```python
from build123d import *

# Parameters (mm, degrees)
SKETCH015_R            = 14.2875
SKETCH015_R_2          = 12.7
PAD015_DEPTH           = 29.21
SKETCH016_R            = 16.66875
SKETCH016_R_2          = 12.7
PAD016_DEPTH           = 12.7
SKETCH014_R            = 3.571875
PAD014_DEPTH           = 13
SKETCH013_R            = 34.925
SKETCH013_R_2          = 14.2875
PAD013_DEPTH           = 12.7
CUT006_PLACEMENT_ANGLE = 60
CUT007_PLACEMENT_ANGLE = 60
CUT008_PLACEMENT_ANGLE = 60
CUT009_PLACEMENT_ANGLE = 60
CUT010_PLACEMENT_ANGLE = 60


with BuildPart() as body015:
    # Sketch015 → Pad015 (new body)
    with BuildSketch(Plane.XZ):
        Circle(SKETCH015_R)
        Circle(SKETCH015_R_2, mode=Mode.SUBTRACT)
    extrude(amount=PAD015_DEPTH)


with BuildPart() as body015_1:
    # Body015 placement: moved
    add(body015.part.moved(Location((0, -0.16, 0))))


with BuildPart() as body016:
    # Sketch016 → Pad016 (new body)
    with BuildSketch(Plane.XZ):
        Circle(SKETCH016_R)
        Circle(SKETCH016_R_2, mode=Mode.SUBTRACT)
    extrude(amount=PAD016_DEPTH)


with BuildPart() as body016_1:
    # Body016 placement: moved
    add(body016.part.moved(Location((0, -29.37, 0))))


with BuildPart() as body014:
    # Sketch014 → Pad014 (new body)
    with BuildSketch(Plane.XZ):
        with Locations((0, 29.36875)):
            Circle(SKETCH014_R)
    extrude(amount=PAD014_DEPTH)


with BuildPart() as fusion001:
    # Sketch013 → Pad013 (new body)
    with BuildSketch(Plane.XZ):
        Circle(SKETCH013_R)
        Circle(SKETCH013_R_2, mode=Mode.SUBTRACT)
    extrude(amount=PAD013_DEPTH)

    # Cut006: cut Body014
    add(body014.part, mode=Mode.SUBTRACT)


with BuildPart() as fusion001_1:
    # Cut006 placement: moved
    add(fusion001.part.rotate(Axis((0, 0, 0), (0, 1, 0)), CUT006_PLACEMENT_ANGLE))

    # Cut007: cut Body014
    add(body014.part, mode=Mode.SUBTRACT)


with BuildPart() as fusion001_2:
    # Cut007 placement: moved
    add(fusion001_1.part.rotate(Axis((0, 0, 0), (0, 1, 0)), CUT007_PLACEMENT_ANGLE))

    # Cut008: cut Body014
    add(body014.part, mode=Mode.SUBTRACT)


with BuildPart() as fusion001_3:
    # Cut008 placement: moved
    add(fusion001_2.part.rotate(Axis((0, 0, 0), (0, 1, 0)), CUT008_PLACEMENT_ANGLE))

    # Cut009: cut Body014
    add(body014.part, mode=Mode.SUBTRACT)


with BuildPart() as fusion001_4:
    # Cut009 placement: moved
    add(fusion001_3.part.rotate(Axis((0, 0, 0), (0, 1, 0)), CUT009_PLACEMENT_ANGLE))

    # Cut010: cut Body014
    add(body014.part, mode=Mode.SUBTRACT)


with BuildPart() as fusion001_5:
    # Cut010 placement: moved
    add(fusion001_4.part.rotate(Axis((0, 0, 0), (0, 1, 0)), CUT010_PLACEMENT_ANGLE))

    # Cut011: cut Body014
    add(body014.part, mode=Mode.SUBTRACT)

    # Fusion001: union Body015, Body016
    add(body015_1.part)
    add(body016_1.part)


solid = fusion001_5.part
```
Source: CAD feature listing. Evaluate the final solid. Frame: model axes, mm. A direction names the side the tool comes from. Round coordinates to 2 decimals unless told otherwise and drop trailing zeros. Loops run counter-clockwise (first coordinate to the right, second up) from the corner with the lowest first, then second, coordinate; pieces in that order, holes last. Notation, with made-up numbers: M 53,6.25 L 107,6.25 A17 ccw 107,36.25 Z; hole C 60.25,86 d11. An arc over 180 degrees is marked long. Put each result on its own line as item: value.
(1) Section C-C, the plane x = -10.5. Return loops of the section in (y, z).
Solutions:
outline: M -42.07,-12.95 L -29.37,-12.95 L -29.37,-9.69 L -12.7,-9.69 L -12.7,-33.31 L 0,-33.31 L 0,-9.69 L -0.16,-9.69 L -0.16,-7.14 L -42.07,-7.14 Z; M -42.07,7.14 L -0.16,7.14 L -0.16,9.69 L 0,9.69 L 0,33.31 L -12.7,33.31 L -12.7,9.69 L -29.37,9.69 L -29.37,12.95 L -42.07,12.95 Z
(2) Pull-direction query (Z, two-part tool) for faces 3 (the face through (13.63, -20.92, 4.29)), 4 (the face through (-13, -0.16, -1)), 5 (the face through (14, -29.37, 5)); classes: released by +Z, released by -Z, zero draft, split by the parting line, or undercut.
Solutions:
face 3: split by the parting line
face 4: undercut
face 5: zero draft
(3) Access query for faces 1 (the face through (-2.75, -20.82, -12.4)), 2 (the face through (15.9, -35.6, 5)). Directions: +Z, -Z, +X, -X, +Y, -Y. A direction counts if a zero-diameter tool reaches every point of the face in a straight line with its end or side. Return the directions, or none.
Solutions:
face 1: +Y, -Y
face 2: -Y
(4) Section D-D, the plane y = -22. Return loops of the section in (x, z) (1 decimal).
Solutions:
outline: C 0,0 d28.6; hole C 0,0 d25.4
(5) Ray query, line 1 (X direction, y = -4, z = 17.5); line 2 (X direction, y = -23, z = 1); line 3 (Y direction, x = -7, z = 20.5). Return the intervals inside material, ascending. Write a range as [from, to].
Solutions:
line 1: [-30.22, -27.63], [-23.24, 23.24], [27.63, 30.22]
line 2: [-14.25, -12.66], [12.66, 14.25]
line 3: [-12.7, 0]
(6) First-contact query: pin 1 (10 mm diameter, centred on x = 6.5, z = -4.5, fed in from +Y); pin 2 (5 mm diameter, centred on x = -12.5, y = -13, fed in from +Z); pin 3 (9.5 mm diameter, centred on x = 0, z = 29.37, fed in from -Y). Flat tips, straight axial feed; report the tip coordinate or a pass-through.
Solutions:
pin 1: y = -0.16
pin 2: z = 33.46
pin 3: y = -12.7
(7) Section A-A, the plane x = 0. State how many separate pieces and enclosed holes the cut face has, and give its area (3 significant figures).
Solutions:
separate pieces: 4
enclosed holes: 0
area: 536 mm²
